from build123d import *

# Parameters (mm, degrees)
SKETCH1_W         = 30
SKETCH1_H         = 30
CENTER_DEPTH      = 25
SKETCH2_W         = 20
SKETCH2_H         = 20
CENTER_HOLE_DEPTH = 20
SKETCH3_W         = 25
SKETCH3_H         = 10
ARM_DEPTH         = 10
SKETCH5_R         = 2.5
SCREW_HOLE_DEPTH  = 48.16990566
SKETCH7_W         = 10
SKETCH7_H         = 10
LEG_DEPTH         = 30
LEG_TAPER         = 5
CIRPATTERN1_COUNT = 4
CHAMFER1_SIZE     = 5
CHAMFER2_SIZE     = 5
CHAMFER3_SIZE     = 5
CHAMFER4_SIZE     = 7
CHAMFER4_SIZE_2   = 0.872143839


with BuildPart() as part:
    # Sketch1 → center (new body)
    with BuildSketch(Plane(origin=(0, 0, 0), x_dir=(1, 0, 0), z_dir=(0, 1, 0))):
        Rectangle(SKETCH1_W, SKETCH1_H)
    extrude(amount=-CENTER_DEPTH)

    # Sketch2 → center hole (cut)
    with BuildSketch(Plane(origin=(0, 0, 0), x_dir=(1, 0, 0), z_dir=(0, 1, 0))):
        Rectangle(SKETCH2_W, SKETCH2_H)
    extrude(amount=-CENTER_HOLE_DEPTH, mode=Mode.SUBTRACT)

    # Sketch3 → arm (add)
    with BuildSketch(Plane(origin=(0, 0, 0), x_dir=(1, 0, 0), z_dir=(0, 1, 0))):
        with Locations((27.5, 0)):
            Rectangle(SKETCH3_W, SKETCH3_H)
    arm = extrude(amount=-ARM_DEPTH)

    # Sketch5 → screw hole (cut, through all)
    with BuildSketch(Plane(origin=(0, -20, 0), x_dir=(1, 0, 0), z_dir=(0, 1, 0))):
        with Locations(Location((0, 0, 0), (0, 0, 270))):
            Circle(SKETCH5_R)
    extrude(amount=-SCREW_HOLE_DEPTH, mode=Mode.SUBTRACT)

    # Sketch7 → leg (add)
    with BuildSketch(Plane.XZ.offset(10)):
        with Locations((35, 0)):
            Rectangle(SKETCH7_W, SKETCH7_H)
    leg = extrude(amount=LEG_DEPTH, taper=LEG_TAPER)

    # CirPattern1: arm, leg ×4 about axis
    cirpattern1_axis = Axis((0, 0, 0), (0, 1, 0))
    add([arm.rotate(cirpattern1_axis, i * 360 / CIRPATTERN1_COUNT) for i in range(1, CIRPATTERN1_COUNT)])
    add([leg.rotate(cirpattern1_axis, i * 360 / CIRPATTERN1_COUNT) for i in range(1, CIRPATTERN1_COUNT)])

    # Chamfer1
    chamfer1_edges = [part.edges().sort_by_distance(p)[0] for p in [
        (15, -12.5, 15),
        (-15, -12.5, 15),
        (-15, -12.5, -15),
        (15, -12.5, -15),
    ]]
    chamfer(chamfer1_edges, length=CHAMFER1_SIZE)

    # Chamfer2
    chamfer2_edges = [part.edges().sort_by_distance(p)[0] for p in [
        (40, 0, 0),
        (0, 0, -40),
        (-40, 0, 0),
        (0, 0, 40),
    ]]
    chamfer(chamfer2_edges, length=CHAMFER2_SIZE)

    # Chamfer3
    chamfer3_edges = [part.edges().sort_by_distance(p)[0] for p in [
        (-15, -25, 0),
        (0, -25, 15),
        (15, -25, 0),
        (0, -25, -15),
        (12.5, -25, 12.5),
        (12.5, -25, -12.5),
        (-12.5, -25, -12.5),
        (-12.5, -25, 12.5),
    ]]
    chamfer(chamfer3_edges, length=CHAMFER3_SIZE)

    # Chamfer4
    # the kernel refuses this chamfer: 7, 0.872143839 mm, written as the material it takes off along each edge
    with BuildSketch(Plane(origin=(-37.375340094, -40, 20.570322389), x_dir=(-0.08715574274765861, 0.9961946980917454, 0), z_dir=(0, 0, -1)), Plane(origin=(-55.570322389, -40, -2.375340094), x_dir=(0, 0.9961946980917455, -0.08715574274765818), z_dir=(1, 0, 0)), Plane(origin=(-32.624659906, -40, -20.570322389), x_dir=(0.08715574274765861, 0.9961946980917454, 0), z_dir=(0, 0, 1)), Plane(origin=(-14.429677611, -40, 2.375340094), x_dir=(0, 0.9961946980917455, 0.08715574274765825), z_dir=(-1, 0, 0)), Plane(origin=(20.570322389, -40, 37.375340094), x_dir=(0, 0.9961946980917454, 0.08715574274765861), z_dir=(-1, 0, 0)), Plane(origin=(-2.375340094, -40, 55.570322389), x_dir=(-0.08715574274765818, 0.9961946980917455, 0), z_dir=(0, 0, -1)), Plane(origin=(-20.570322389, -40, 32.624659906), x_dir=(0, 0.9961946980917454, -0.08715574274765861), z_dir=(1, 0, 0)), Plane(origin=(2.375340094, -40, 14.429677611), x_dir=(0.08715574274765818, 0.9961946980917455, 0), z_dir=(0, 0, 1)), Plane(origin=(37.375340094, -40, -20.570322389), x_dir=(0.08715574274765861, 0.9961946980917454, 0), z_dir=(0, 0, 1)), Plane(origin=(55.570322389, -40, 2.375340094), x_dir=(0, 0.9961946980917455, 0.08715574274765825), z_dir=(-1, 0, 0)), Plane(origin=(32.624659906, -40, 20.570322389), x_dir=(-0.08715574274765861, 0.9961946980917454, 0), z_dir=(0, 0, -1)), Plane(origin=(14.429677611, -40, -2.375340094), x_dir=(0, 0.9961946980917455, -0.08715574274765825), z_dir=(1, 0, 0)), Plane(origin=(-20.570322389, -40, -37.375340094), x_dir=(0, 0.9961946980917454, -0.08715574274765861), z_dir=(1, 0, 0)), Plane(origin=(2.375340094, -40, -55.570322389), x_dir=(0.08715574274765818, 0.9961946980917455, 0), z_dir=(0, 0, 1)), Plane(origin=(20.570322389, -40, -32.624659906), x_dir=(0, 0.9961946980917454, 0.08715574274765861), z_dir=(-1, 0, 0)), Plane(origin=(-2.375340094, -40, -14.429677611), x_dir=(-0.08715574274765818, 0.9961946980917455, 0), z_dir=(0, 0, -1))) as chamfer4_piece_1:
        Polygon((CHAMFER4_SIZE, 0), (-CHAMFER4_SIZE_2 * 0.0871557427705, CHAMFER4_SIZE_2 * 0.996194698353), (0, 0), align=None)
    extrude(amount=41.140644778, mode=Mode.SUBTRACT)


solid = part.part
Design review of the part built by this model. Coordinates are the model's own, in mm. A direction names the side the tool comes from. Give positions to 0.01 mm unless a question says otherwise; leave off trailing zeros. Order: outer loops, then holes, each group sorted by start corner. A loop starts at its lowest first (then second) coordinate and runs counter-clockwise, first axis right, second up.
1. Mouldability with a two-part tool opening along Z and no side actions: class faces 4 (the flat face through (0, -7, 40)), 5 (the flat face through (22, -10, 0)), 6 (the flat face through (-35.04, -35.69, -2.42)), 7 (the flat face through (0, -10, 22)) as +Z half, -Z half, draft (parallel to the pull), parting line (faces both ways), or undercut.
Solution:
face 4: +Z half
face 5: draft
face 6: -Z half
face 7: undercut
2. Add section A-A, the plane y = -11. State how many separate pieces and enclosed holes the cut face has, then the cut area to 3 significant figures.
Solution:
separate pieces: 5
enclosed holes: 1
area: 836 mm2
3. To check wall thickness, follow L1, parallel to X at y = -22.7, z = 0; L2, parallel to X at y = -7, z = 8.5; L3, parallel to X at y = -22.5, z = 0. State the ranges of each line that lie inside material, in increasing order.
Solution:
L1: x = -38.89 to -31.11, -12.3 to -2.5, 2.5 to 12.3, 31.11 to 38.89
L2: x = -15 to -10, 10 to 15
L3: x = -38.91 to -31.09, -12.5 to -2.5, 2.5 to 12.5, 31.09 to 38.91
4. Add section B-B, the plane x = 25. State the section outline as (y, z) points, then the cut area to 3 significant figures.
Solution:
outline: (-10, -5) - (0, -5) - (0, 5) - (-10, 5) - close
area: 100 mm2
5. Add section C-C, the plane z = -28. State the section outline as (x, y) points, then the cut area to 3 significant figures.
Solution:
outline: (-5, -10) - (5, -10) - (5, 0) - (-5, 0) - close
area: 100 mm2
6. For pin 1 Ø8 at (x, z) = (17.5, -18) entering from -Y; pin 2 Ø16 at (x, z) = (-4.5, 3) entering from +Y; pin 3 Ø3 at (y, z) = (-5, 26) entering from -X; pin 4 Ø5 at (y, z) = (-6, -28.5) entering from +X, all flat-tipped, find the tip position at first contact; note any pin that passes through.
Solution:
pin 1: passes through
pin 2: stops at y = 0
pin 3: stops at x = -5
pin 4: stops at x = 5
7. Tool access review of faces 1 (the flat face through (-27, -5, -5)), 2 (the flat face through (15, -12, 0)), 3 (the flat face through (-32.58, -35.69, -0.04)): name each direction out of +Z, -Z, +X, -X, +Y, -Y from which nothing blocks a thin tool from reaching the whole face with its end or side.
Solution:
face 1: -Z, -X, +Y, -Y
face 2: -Y
face 3: +Z, -Z, -Y
